For this review, take the finished solid that the model builds, in its own axes (mm). Face numbers are marked on the shaded views. Round coordinates to 2 decimals unless told otherwise and drop trailing zeros. Loops run counter-clockwise (first coordinate to the right, second up) from the corner with the lowest first, then second, coordinate; pieces in that order, holes last.
1) Take a section at C-C (y = 1.5). State the section outline as (x, z) points.
2) Take a section at B-B (x = 12). State the section outline as (y, z) points, then the cut area to 3 significant figures.
3) Mouldability with a two-part tool opening along Y and no side actions: class the marked faces 1, 2, 3 and 4 as pulls with the +Y half, pulls with the -Y half, needs draft (parallel to the pull), parting line crosses it, or undercut.
4) Insertion check: pin 1 (0.6 mm diameter, centred on x = 2, y = 29, fed in from +Z); pin 2 (6 mm diameter, centred on x = 13.5, y = 22.5, fed in from -Z). Each pin has a flat end and moves straight along its axis. Give the tip position at first contact, or say it passes through.
5) Wall thickness on L1, parallel to Y at x = -3, z = 18.75; L2, parallel to X at y = -20, z = 8; L3, parallel to Z at x = -4.5, y = -11: over which ranges is each line inside the solid? List them lowest first.
6) Take a section at A-A (z = 15.25). State the section outline as (x, y) points.
```python
from build123d import *

# Parameters (mm, degrees)
F0_W     = 35
F0_H     = 60
F1_DEPTH = 30
F2_W     = 31
F2_H     = 56
F3_DEPTH = 28
F4_W     = 5
F4_H     = 8
F4_W_2   = 10
F5_DEPTH = 2
F6_W     = 7
F6_H     = 8
F7_DEPTH = 2


with BuildPart() as f1:
    # F0 (on Top) → F1 (new body)
    with BuildSketch(Plane.XY):
        Rectangle(F0_W, F0_H)
    extrude(amount=F1_DEPTH)

    # F2 (on face) → F3 (cut)
    with BuildSketch(Plane.XY.offset(30)):
        Rectangle(F2_W, F2_H)
    extrude(amount=-F3_DEPTH, mode=Mode.SUBTRACT)

    # F4 (on face) → F5 (cut)
    with BuildSketch(Plane(origin=(0, 30, 0), x_dir=(-1, 0, 0), z_dir=(0, 1, 0))):
        with Locations((2.5, 26)):
            Rectangle(F4_W, F4_H)
        with Locations((-5, 26)):
            Rectangle(F4_W_2, F4_H)
    extrude(amount=-F5_DEPTH, mode=Mode.SUBTRACT)

    # F6 (on face) → F7 (cut)
    with BuildSketch(Plane.XZ.offset(30)):
        with Locations((-3.5, 26)):
            Rectangle(F6_W, F6_H)
        with Locations((3.5, 26)):
            Rectangle(F6_W, F6_H)
    extrude(amount=-F7_DEPTH, mode=Mode.SUBTRACT)


solid = f1.part
```
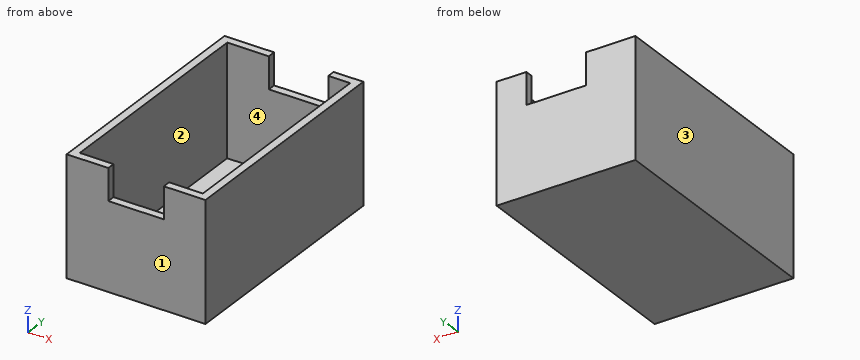
Response:
1. outline: (-17.5, 0) - (17.5, 0) - (17.5, 30) - (15.5, 30) - (15.5, 2) - (-15.5, 2) - (-15.5, 30) - (-17.5, 30) - close
2. outline: (-30, 0) - (30, 0) - (30, 30) - (28, 30) - (28, 2) - (-28, 2) - (-28, 30) - (-30, 30) - close
2. area: 232 mm2
3. face 1: pulls with the -Y half
3. face 2: undercut
3. face 3: needs draft
3. face 4: undercut
4. pin 1: stops at z = 22
4. pin 2: stops at z = 0
5. L1: y = -30 to -28, 28 to 30
5. L2: x = -17.5 to -15.5, 15.5 to 17.5
5. L3: z = 0 to 2
6. outline: (-17.5, -30) - (17.5, -30) - (17.5, 30) - (-17.5, 30) - close; hole (-15.5, -28) - (15.5, -28) - (15.5, 28) - (-15.5, 28) - close
